The listing builds one solid part. Answer for the finished solid, in the listing's coordinates (mm). A direction names the side the tool comes from. Coordinates: 2 decimals unless noted, no trailing zeros. Write each loop counter-clockwise with the first axis right and the second up, starting at its lowest first coordinate (ties: lowest second). Pieces come first, ordered by that corner, then holes. Notation, with made-up numbers: M -5.75,75 L 15.25,75 A13 cw 15.25,79 Z; hole C -38,37 d1. An arc over 180 degrees is marked long. Answer as CSV lines item,"result".
```python
from build123d import *

# Parameters (mm, degrees)
BOSS_EXTRUDE1_DEPTH       = 15
BOSS_EXTRUDE2_DEPTH       = 2.85
SKETCH4_W                 = 1.05
SKETCH4_H                 = 0.3
REVOLVE1_ANGLE            = 180
SKETCH5_R                 = 1.9
BOSS_EXTRUDE3_DEPTH       = 6
BOSS_EXTRUDE4_REACH       = 29.869
BOSS_EXTRUDE4_END_RADIUS  = 6
SKETCH6_W                 = 6
SKETCH6_H                 = 8
SKETCH8_W                 = 1.75
SKETCH8_H                 = 3
REVOLVE2_ANGLE            = 90
BOSS_EXTRUDE5_DEPTH       = 15
BOSS_EXTRUDE5_START       = -8
BOSS_EXTRUDE5_2_OUTLINE_R = 1.9
BOSS_EXTRUDE5_2_DEPTH     = 2


with BuildPart() as part:
    # Sketch1 → Boss-Extrude1 (new body)
    with BuildSketch(Plane.XY):
        with BuildLine():
            Line((0, -5), (0, -14.5))
            Line((0, -14.5), (-6, -14.5))
            Line((-6, -14.5), (-6, 0))
            ThreePointArc((-6, 0), (-4.242640687, 4.242640687), (0, 6))
            Line((0, 6), (0, 5))
            ThreePointArc((0, 5), (-5, 0), (0, -5))
        make_face()
    extrude(amount=BOSS_EXTRUDE1_DEPTH)

    # Sketch3 → Boss-Extrude2 (add)
    with BuildSketch(Plane(origin=(-6, 0, 0), x_dir=(0, 0, -1), z_dir=(1, 0, 0))):
        with BuildLine():
            Line((1.5, -8.35), (0, -8.35))
            Line((0, -8.35), (0, -11.15))
            Line((0, -11.15), (1.5, -11.15))
            ThreePointArc((1.5, -11.15), (2.9, -9.75), (1.5, -8.35))
        make_face()
        with BuildLine():
            Line((-16.5, -11.15), (-15, -11.15))
            Line((-15, -11.15), (-15, -8.35))
            Line((-15, -8.35), (-16.5, -8.35))
            ThreePointArc((-16.5, -8.35), (-17.9, -9.75), (-16.5, -11.15))
        make_face()
    extrude(amount=BOSS_EXTRUDE2_DEPTH)

    # Sketch4 → Revolve1 (revolve)
    with BuildSketch(Plane(origin=(0, 0, 0), x_dir=(0, 0, -1), z_dir=(1, 0, 0))):
        with Locations((-11.575, 4.85)):
            Rectangle(SKETCH4_W, SKETCH4_H)
        with Locations((-3.425, 4.85)):
            Rectangle(SKETCH4_W, SKETCH4_H)
    revolve(axis=Axis((0, 0, 15), (0, 0, 1)), revolution_arc=REVOLVE1_ANGLE)



with BuildPart() as body_2:
    # Sketch5 → Boss-Extrude3 (new body)
    with BuildSketch(Plane(origin=(0, 0, 0), x_dir=(0, 0, -1), z_dir=(1, 0, 0))):
        with BuildLine():
            Line((-11.5, 6), (-11.5, 10.2))
            ThreePointArc((-11.5, 10.2), (-7.5, 14.2), (-3.5, 10.2))
            Line((-3.5, 10.2), (-3.5, 6))
            Line((-3.5, 6), (-11.5, 6))
        make_face()
        with Locations((-7.5, 10.2)):
            Circle(SKETCH5_R, mode=Mode.SUBTRACT)
    extrude(amount=-BOSS_EXTRUDE3_DEPTH)


with BuildPart() as part_1:
    add(part.part)

    add(body_2.part)  # Boss-Extrude4 merges body 2
    # Boss-Extrude4: up to this cylinder (the profile starts outside it)
    boss_extrude4_end = Plane(origin=(0, 0, 7.5), z_dir=(0, 0, -1)) * Cylinder(BOSS_EXTRUDE4_END_RADIUS, 72.738, mode=Mode.PRIVATE)
    # Sketch6 → Boss-Extrude4 (add, up to the surface)
    with BuildSketch(Plane.XZ.offset(-6), mode=Mode.PRIVATE) as boss_extrude4_sk1:
        with Locations((-3, 7.5)):
            Rectangle(SKETCH6_W, SKETCH6_H)
    boss_extrude4_tool1 = extrude(boss_extrude4_sk1.sketch, amount=BOSS_EXTRUDE4_REACH, mode=Mode.PRIVATE) - boss_extrude4_end
    add(boss_extrude4_tool1.solids().sort_by_distance((-3, 6, 7.5))[0])

    # Sketch7 → Cut-Revolve1 (revolve, cut)
    with BuildSketch(Plane(origin=(0, 0, 0), x_dir=(0, 0, -1), z_dir=(1, 0, 0))):
        Polygon((-15, 5.2), (-15, 5), (-12.1, 5), (-12.1, 4.7), (-11.05, 4.7), (-11.05, 5), (-3.95, 5), (-3.95, 4.7), (-2.9, 4.7), (-2.9, 5), (0, 5), (0, 5.2), align=None)
    revolve(axis=Axis((0, 0, 15), (0, 0, -1)), mode=Mode.SUBTRACT)

    # Sketch8 → Revolve2 (revolve)
    with BuildSketch(Plane(origin=(0, 0, 0), x_dir=(0, 0, -1), z_dir=(1, 0, 0))):
        with Locations((-15.875, 4.5)):
            Rectangle(SKETCH8_W, SKETCH8_H)
        with Locations((0.875, 4.5)):
            Rectangle(SKETCH8_W, SKETCH8_H)
    revolve(axis=Axis((0, 0, 15), (0, 0, 1)), revolution_arc=REVOLVE2_ANGLE)

    # Boss-Extrude5: read off the stored shape, not the designer's step
    # Boss-Extrude5 outline → Boss-Extrude5 (add)
    with BuildSketch(Plane.XY):
        with BuildLine():
            Line((-8, -14.5), (-6, -14.5))
            Line((-6, -14.5), (-6, 0))
            ThreePointArc((-6, 0), (-4.242640687, 4.242640687), (0, 6))
            Line((0, 6), (-8, 6))
            Line((-8, 6), (-8, -14.5))
        make_face()
    extrude(amount=BOSS_EXTRUDE5_DEPTH)

    # Boss-Extrude5 2 outline → Boss-Extrude5 2 (add)
    with BuildSketch(Plane.YZ.offset(BOSS_EXTRUDE5_START)):
        with BuildLine():
            Line((10.2, 11.5), (6, 11.5))
            Line((6, 11.5), (6, 3.5))
            Line((6, 3.5), (10.2, 3.5))
            ThreePointArc((10.2, 3.5), (14.2, 7.5), (10.2, 11.5))
        make_face()
        with Locations((10.2, 7.5)):
            Circle(BOSS_EXTRUDE5_2_OUTLINE_R, mode=Mode.SUBTRACT)
    extrude(amount=BOSS_EXTRUDE5_2_DEPTH)


solid = part_1.part
```
Q1. Find section B-B (z = 7.5). Give the vertices of the cut face in (x, y), and give its area (3 significant figures).
Output:
outline,"M -8,-14.5 L 0,-14.5 L 0,-5.2 A5.2 cw 0,5.2 L 0,8.3 L -8,8.3 Z; M -8,12.1 L 0,12.1 L 0,14.2 L -8,14.2 Z"
area,"157 mm2"
Q2. Flat-ended cylindrical pins translate along their axes: pin 1 Ø4 at (x, y) = (-1.5, 11) entering from +Z; pin 2 Ø1.6 at (x, z) = (-4.5, -1) entering from +Y; pin 3 Ø4 at (x, z) = (-3.5, 1) entering from +Y. Find the tip coordinate at first contact, or state that the pin passes through.
Output:
pin 1,"z = 11.5"
pin 2,"y = 4.72"
pin 3,"y = 6"
Q3. Find section D-D (z = 12.5). Give the vertices of the cut face in (x, y).
Output:
outline,"M -8,-14.5 L 0,-14.5 L 0,-5.2 A5.2 cw 0,5.2 L 0,6 L -8,6 Z"
Q4. Straight lines are drawn through the part: line 1 (Z direction, x = -6.7, y = 10.2); line 2 (Y direction, x = -4, z = 6); line 3 (Y direction, x = -7.2, z = 7.5). For each, find the intervals that lie inside material, in ascending order.
Output:
line 1,"3.5 to 5.6, 9.4 to 11.5"
line 2,"-14.5 to -3.32, 3.32 to 9.03, 11.37 to 13.91"
line 3,"-14.5 to 8.3, 12.1 to 14.2"
Q5. For faces 5 (the flat face through (-5, 0, -1)), 6 (the flat face through (-5, 0, 16)), 7 (the flat face through (-6, -10, 16)), 8 (the flat face through (-3, 3, 15)), determine the directions among +Z, -Z, +X, -X, +Y, -Y from which every point of the face is accessible in a straight line to the end or side of a thin tool.
Output:
face 5,"-Z, +X, -X"
face 6,"+Z, +X, -X"
face 7,"+Z, -X, +Y, -Y"
face 8,"+X"
Q6. Find section A-A (x = -1.25). Give the vertices of the cut face in (y, z).
Output:
outline,"M -14.5,0 L -5.05,0 L -5.05,15 L -14.5,15 Z; M 2.73,-1.75 L 5.87,-1.75 L 5.87,0 L 6,0 L 6,3.5 L 10.2,3.5 A4 ccw 10.2,11.5 L 6,11.5 L 6,15 L 5.87,15 L 5.87,16.75 L 2.73,16.75 L 2.73,15 L 5.05,15 L 5.05,0 L 2.73,0 Z; hole C 10.2,7.5 d3.8"
Q7. The mould has two halves that part along Y. Classify faces 1 (the cylindrical face through (-4.196, 4.289, -0.887)), 2 (the flat face through (-3, 3, 0)), 3 (the flat face through (-4, 8, 11.5)), 4 (the cylindrical face through (-5.2, -0.1, 7.6)): pulls with the +Y half, pulls with the -Y half, needs draft (parallel to the pull), parting line crosses it, or undercut.
Output:
face 1,"pulls with the +Y half"
face 2,"undercut"
face 3,"needs draft"
face 4,"undercut"
Q8. Find section C-C (y = 2). Give the vertices of the cut face in (x, z).
Output:
outline,"M -8,0 L -5.66,0 L -5.66,-1.75 L -2.24,-1.75 L -2.24,0 L -4.8,0 L -4.8,15 L -2.24,15 L -2.24,16.75 L -5.66,16.75 L -5.66,15 L -8,15 Z"
